Read the model definition and answer for the solid it produces. Units are mm, in the model's axes. A direction names the side the tool comes from. Coordinates: 2 decimals unless noted, no trailing zeros. Write each loop counter-clockwise with the first axis right and the second up, starting at its lowest first coordinate (ties: lowest second). Pieces come first, ordered by that corner, then holes. Notation, with made-up numbers: (44, 6) -> (52, 6) arc R27 ccw to (52, 40) -> close; hole circle Ø4 at (11.5, 81). An arc over 180 degrees is marked (long way). Return JSON: item names as keys, results as strings.
from build123d import *

# Parameters (mm, degrees)
SKETCH1_W           = 33.5
SKETCH1_H           = 25
SKETCH1_W_2         = 29.5
SKETCH1_H_2         = 21
BOSS_EXTRUDE1_DEPTH = 2
SKETCH1_3_W         = 33.5
SKETCH1_3_H         = 25
SKETCH1_3_W_2       = 29.5
SKETCH1_3_H_2       = 21
BOSS_EXTRUDE2_DEPTH = 25
SKETCH2_W           = 2
SKETCH2_H           = 8
CUT_EXTRUDE1_DEPTH  = 20
SKETCH3_W           = 2
SKETCH3_H           = 2
BOSS_EXTRUDE3_DEPTH = 5
CHAMFER1_SIZE       = 2
CUT_EXTRUDE2_DEPTH  = 5


with BuildPart() as part:
    # Sketch1 → Boss-Extrude1 (new body)
    # profile 1 of 2: a face of its own
    with BuildSketch(Plane(origin=(0, 0, 0), x_dir=(1, 0, 0), z_dir=(0, 1, 0))):
        with Locations((5.204545455, 5.939393939)):
            Rectangle(SKETCH1_W, SKETCH1_H)
        with Locations((5.204545455, 5.939393939)):
            Rectangle(SKETCH1_W_2, SKETCH1_H_2, mode=Mode.SUBTRACT)
    # profile 2 of 2: a face of its own
    with BuildSketch(Plane(origin=(0, 0, 0), x_dir=(1, 0, 0), z_dir=(0, 1, 0))):
        with Locations((5.204545455, 5.939393939)):
            Rectangle(SKETCH1_W_2, SKETCH1_H_2)
    extrude(amount=BOSS_EXTRUDE1_DEPTH)

    # Sketch1<3> → Boss-Extrude2 (add)
    with BuildSketch(Plane(origin=(0, 0, 0), x_dir=(1, 0, 0), z_dir=(0, 1, 0))):
        with Locations((5.204545455, 5.939393939)):
            Rectangle(SKETCH1_3_W, SKETCH1_3_H)
        with Locations((5.204545455, 5.939393939)):
            Rectangle(SKETCH1_3_W_2, SKETCH1_3_H_2, mode=Mode.SUBTRACT)
    extrude(amount=BOSS_EXTRUDE2_DEPTH)

    # Sketch2 → Cut-Extrude1 (cut)
    with BuildSketch(Plane(origin=(0, 25, 0), x_dir=(1, 0, 0), z_dir=(0, 1, 0))):
        with Locations((20.954545455, 7.439393939)):
            Rectangle(SKETCH2_W, SKETCH2_H)
    extrude(amount=-CUT_EXTRUDE1_DEPTH, mode=Mode.SUBTRACT)

    # Sketch3 → Boss-Extrude3 (add)
    with BuildSketch(Plane(origin=(0, 25, 0), x_dir=(1, 0, 0), z_dir=(0, 1, 0))):
        with Locations((-8.545454545, 15.439393939)):
            Rectangle(SKETCH3_W, SKETCH3_H)
        with Locations((-8.545454545, -3.560606061)):
            Rectangle(SKETCH3_W, SKETCH3_H)
        with Locations((18.954545455, -3.560606061)):
            Rectangle(SKETCH3_W, SKETCH3_H)
        with Locations((18.954545455, 15.439393939)):
            Rectangle(SKETCH3_W, SKETCH3_H)
    extrude(amount=-BOSS_EXTRUDE3_DEPTH)

    # Chamfer1
    chamfer1_edges = [part.edges().sort_by_distance(p)[0] for p in [
        (18.954545455, 20, 4.560606061),
        (-8.545454545, 20, 4.560606061),
        (18.954545455, 20, -16.439393939),
        (-8.545454545, 20, -16.439393939),
    ]]
    chamfer(chamfer1_edges, length=CHAMFER1_SIZE - 0.0001)  # a hair under: the kernel refuses the full size

    # Sketch4 → Cut-Extrude2 (cut)
    with BuildSketch(Plane(origin=(0, 25, 0), x_dir=(1, 0, 0), z_dir=(0, 1, 0))):
        with BuildLine():
            ThreePointArc((20.454545455, -4.560606061), (20.308098845, -4.20705267), (19.954545455, -4.060606061))
            Line((19.954545455, -4.060606061), (19.954545455, -4.560606061))
            Line((19.954545455, -4.560606061), (19.454545455, -4.560606061))
            ThreePointArc((19.454545455, -4.560606061), (19.954545455, -5.060606061), (20.454545455, -4.560606061))
        make_face()
        with BuildLine():
            Line((19.954545455, -4.560606061), (19.954545455, -4.060606061))
            ThreePointArc((19.954545455, -4.060606061), (19.600992064, -4.20705267), (19.454545455, -4.560606061))
            Line((19.454545455, -4.560606061), (19.954545455, -4.560606061))
        make_face()
        with BuildLine():
            ThreePointArc((20.454545455, -4.560606061), (20.308098845, -4.20705267), (19.954545455, -4.060606061))
            Line((19.954545455, -4.060606061), (19.954545455, -4.560606061))
            Line((19.954545455, -4.560606061), (19.454545455, -4.560606061))
            ThreePointArc((19.454545455, -4.560606061), (19.954545455, -5.060606061), (20.454545455, -4.560606061))
        make_face()
        with BuildLine():
            Line((19.954545455, -4.560606061), (19.954545455, -4.060606061))
            ThreePointArc((19.954545455, -4.060606061), (19.600992064, -4.20705267), (19.454545455, -4.560606061))
            Line((19.454545455, -4.560606061), (19.954545455, -4.560606061))
        make_face()
        with BuildLine():
            ThreePointArc((20.454545455, 16.439393939), (19.954545455, 16.939393939), (19.454545455, 16.439393939))
            Line((19.454545455, 16.439393939), (19.954545455, 16.439393939))
            Line((19.954545455, 16.439393939), (19.954545455, 15.939393939))
            ThreePointArc((19.954545455, 15.939393939), (20.308098845, 16.085840549), (20.454545455, 16.439393939))
        make_face()
        with BuildLine():
            Line((19.954545455, 16.439393939), (19.454545455, 16.439393939))
            ThreePointArc((19.454545455, 16.439393939), (19.600992064, 16.085840549), (19.954545455, 15.939393939))
            Line((19.954545455, 15.939393939), (19.954545455, 16.439393939))
        make_face()
        with BuildLine():
            ThreePointArc((20.454545455, 16.439393939), (19.954545455, 16.939393939), (19.454545455, 16.439393939))
            Line((19.454545455, 16.439393939), (19.954545455, 16.439393939))
            Line((19.954545455, 16.439393939), (19.954545455, 15.939393939))
            ThreePointArc((19.954545455, 15.939393939), (20.308098845, 16.085840549), (20.454545455, 16.439393939))
        make_face()
        with BuildLine():
            Line((19.954545455, 16.439393939), (19.454545455, 16.439393939))
            ThreePointArc((19.454545455, 16.439393939), (19.600992064, 16.085840549), (19.954545455, 15.939393939))
            Line((19.954545455, 15.939393939), (19.954545455, 16.439393939))
        make_face()
        with BuildLine():
            ThreePointArc((-9.545454545, 15.939393939), (-9.191901155, 16.085840549), (-9.045454545, 16.439393939))
            Line((-9.045454545, 16.439393939), (-9.545454545, 16.439393939))
            Line((-9.545454545, 16.439393939), (-9.545454545, 15.939393939))
        make_face()
        with BuildLine():
            Line((-9.545454545, 16.439393939), (-9.045454545, 16.439393939))
            ThreePointArc((-9.045454545, 16.439393939), (-9.899007936, 16.79294733), (-9.545454545, 15.939393939))
            Line((-9.545454545, 15.939393939), (-9.545454545, 16.439393939))
        make_face()
        with BuildLine():
            ThreePointArc((-9.545454545, 15.939393939), (-9.191901155, 16.085840549), (-9.045454545, 16.439393939))
            Line((-9.045454545, 16.439393939), (-9.545454545, 16.439393939))
            Line((-9.545454545, 16.439393939), (-9.545454545, 15.939393939))
        make_face()
        with BuildLine():
            Line((-9.545454545, 16.439393939), (-9.045454545, 16.439393939))
            ThreePointArc((-9.045454545, 16.439393939), (-9.899007936, 16.79294733), (-9.545454545, 15.939393939))
            Line((-9.545454545, 15.939393939), (-9.545454545, 16.439393939))
        make_face()
        with BuildLine():
            ThreePointArc((-9.045454545, -4.560606061), (-9.191901155, -4.20705267), (-9.545454545, -4.060606061))
            Line((-9.545454545, -4.060606061), (-9.545454545, -4.560606061))
            Line((-9.545454545, -4.560606061), (-9.045454545, -4.560606061))
        make_face()
        with BuildLine():
            Line((-9.545454545, -4.560606061), (-9.545454545, -4.060606061))
            ThreePointArc((-9.545454545, -4.060606061), (-9.899007936, -4.914159451), (-9.045454545, -4.560606061))
            Line((-9.045454545, -4.560606061), (-9.545454545, -4.560606061))
        make_face()
        with BuildLine():
            ThreePointArc((-9.045454545, -4.560606061), (-9.191901155, -4.20705267), (-9.545454545, -4.060606061))
            Line((-9.545454545, -4.060606061), (-9.545454545, -4.560606061))
            Line((-9.545454545, -4.560606061), (-9.045454545, -4.560606061))
        make_face()
        with BuildLine():
            Line((-9.545454545, -4.560606061), (-9.545454545, -4.060606061))
            ThreePointArc((-9.545454545, -4.060606061), (-9.899007936, -4.914159451), (-9.045454545, -4.560606061))
            Line((-9.045454545, -4.560606061), (-9.545454545, -4.560606061))
        make_face()
    extrude(amount=-CUT_EXTRUDE2_DEPTH, mode=Mode.SUBTRACT)


solid = part.part
1. The part is cut by section C-C (z = -2.25). Determine the outline of the cut face in (x, y).
Taken from the geometry:
{"outline": "(-11.55, 0) -> (21.95, 0) -> (21.95, 25) -> (19.95, 25) -> (19.95, 2) -> (-9.55, 2) -> (-9.55, 25) -> (-11.55, 25) -> close"}
2. The part is cut by section A-A (y = 17). Determine the outline of the cut face in (x, z), then the cut area to 3 significant figures.
Taken from the geometry:
{"outline": "(-11.55, -18.44) -> (21.95, -18.44) -> (21.95, -11.44) -> (19.95, -11.44) -> (19.95, -16.44) -> (-9.55, -16.44) -> (-9.55, 4.56) -> (19.95, 4.56) -> (19.95, -3.44) -> (21.95, -3.44) -> (21.95, 6.56) -> (-11.55, 6.56) -> close", "area": "202 mm2"}
3. A tool of negligible diameter and unlimited length cuts with its end or side. For faces 4 (the face through (-9, 23, -14.439)), 5 (the face through (21, 15, -3.439)), 6 (the face through (-8.56, 18.99, 3.57)), from which of +Z, -Z, +X, -X, +Y, -Y can it reach the whole face along a straight path? Write none if from no direction.
Taken from the geometry:
{"face 4": "+Y", "face 5": "+X, +Y", "face 6": "none"}
4. The part is cut by section B-B (x = -6). Determine the outline of the cut face in (y, z), then the cut area to 3 significant figures.
Taken from the geometry:
{"outline": "(0, -18.44) -> (25, -18.44) -> (25, -16.44) -> (2, -16.44) -> (2, 4.56) -> (25, 4.56) -> (25, 6.56) -> (0, 6.56) -> close", "area": "142 mm2"}
5. For a pull along Z with two mould halves and no side action, classify faces 1 (the face through (5, 13, 4.561)), 2 (the face through (5, 0, -6)), 3 (the face through (5, 2, -6)) as +Z half, -Z half, draft (parallel to the pull), parting line (faces both ways), or undercut.
Taken from the geometry:
{"face 1": "undercut", "face 2": "draft", "face 3": "undercut"}
6. A flat-ended cylindrical pin translates along its axis: pin 1 Ø6.5 at (x, z) = (2.5, -4.5) entering from +Y. Find the tip coordinate at first contact, or state that the pin passes through.
Taken from the geometry:
{"pin 1": "stops at y = 2"}
7. Consider L1, parallel to X at y = 14.25, z = -14; L2, parallel to Z at x = 6, y = 15.5; L3, parallel to Z at x = -9, y = 23. Determine where each line is inside the solid, lowest interval first.
Taken from the geometry:
{"L1": "x = -11.55 to -9.55, 19.95 to 21.95", "L2": "z = -18.44 to -16.44, 4.56 to 6.56", "L3": "z = -18.44 to -14.44, 2.56 to 6.56"}
